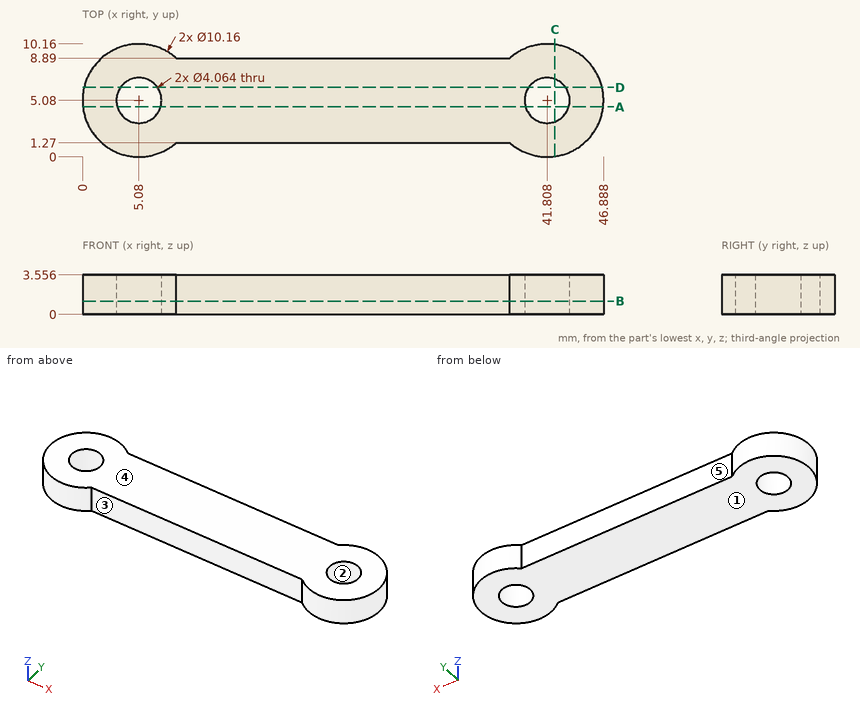
Verification items for this drawing (mm, ordinates from the low corner). A direction names the side the tool comes from. Give positions to 0.01 mm unless a question says otherwise; leave off trailing zeros. Loops run counter-clockwise (first coordinate to the right, second up) from the corner with the lowest first, then second, coordinate; pieces in that order, holes last.
1. Tool access check on the marked faces 3, 4 and 5. Record the directions out of +Z, -Z, +X, -X, +Y, -Y that give a thin tool (end or side, any length) a straight path to the whole face; none if there is none.
Derived:
face 3: +Z, -Z, -Y
face 4: +Z, +X, -X, +Y, -Y
face 5: +Z, -Z, +Y
2. Cross-section at D-D on y = 6.25. Record the cut outline in (x, z).
Derived:
outline: (0.14, 0) - (3.42, 0) - (3.42, 3.56) - (0.14, 3.56) - close; (6.74, 0) - (40.15, 0) - (40.15, 3.56) - (6.74, 3.56) - close; (43.47, 0) - (46.75, 0) - (46.75, 3.56) - (43.47, 3.56) - close
3. Cross-section at C-C on x = 42.5. Record the cut outline in (y, z), and give its area (3 significant figures).
Derived:
outline: (0.05, 0) - (3.17, 0) - (3.17, 3.56) - (0.05, 3.56) - close; (6.99, 0) - (10.11, 0) - (10.11, 3.56) - (6.99, 3.56) - close
area: 22.2 mm2
4. Go/stop test with flat-tipped pins: P1, Ø1.8, axis at x = 25, z = 1, coming from the -Y side; P2, Ø5.5, axis at x = 5.08, y = 5.08, coming from the +Z side; P3, Ø1, axis at y = 8.5, z = 3, coming from the +X side (1 decimal); P4, Ø1.5, axis at y = 7.5, z = 1, coming from the +X side. Record where each tip stops, or that it passes through.
Derived:
P1: stops at y = 1.27
P2: stops at z = 3.56
P3: stops at x = 46
P4: stops at x = 46.61
5. Cross-section at A-A on y = 4.5. Record the cut outline in (x, z) (1 decimal), and give its area (3 significant figures).
Derived:
outline: (0, 0) - (3.1, 0) - (3.1, 3.6) - (0, 3.6) - close; (7, 0) - (39.9, 0) - (39.9, 3.6) - (7, 3.6) - close; (43.8, 0) - (46.9, 0) - (46.9, 3.6) - (43.8, 3.6) - close
area: 139 mm2
6. Cross-section at B-B on z = 1.2. Record the cut outline in (x, y), and give its area (3 significant figures).
Derived:
outline: (8.44, 1.27) - (38.45, 1.27) arc R5.08 ccw (long way) to (38.45, 8.89) - (8.44, 8.89) arc R5.08 ccw (long way) to start; hole circle Ø4.06 at (5.08, 5.08); hole circle Ø4.06 at (41.81, 5.08)
area: 347 mm2
7. Material ranges on probe 1 along X at (y, z) = (6.5, 0.65) (1 decimal); probe 2 along X at (y, z) = (5.5, 0.95); probe 3 along Y at (x, z) = (34, 0.35), recorded low to high.
Derived:
probe 1: x = 0.2 to 3.6, 6.5 to 40.4, 43.3 to 46.7
probe 2: x = 0.02 to 3.09, 7.07 to 39.82, 43.8 to 46.87
probe 3: y = 1.27 to 8.89
8. Release check for a two-part mould opening along X. For the marked faces 1 and 2 record: +X half, -X half, draft (parallel to the pull), parting line (faces both ways), or undercut.
Derived:
face 1: draft
face 2: undercut
